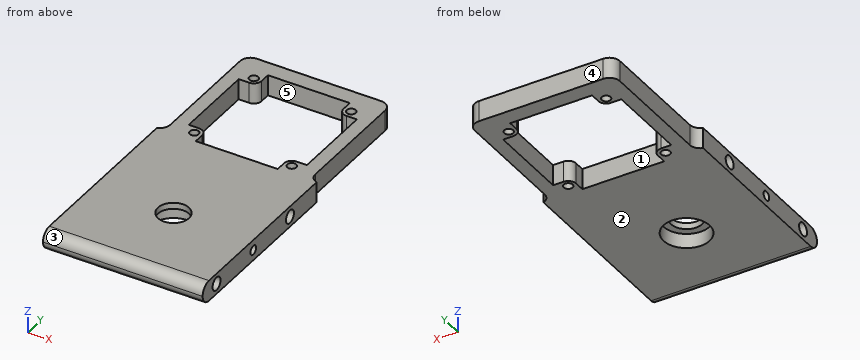
from build123d import *

# Parameters (mm, degrees)
AUFSATZ_LINEAR_AUSTRAGEN1_DEPTH  = 5
SKIZZE2_R                        = 3.15
SCHNITT_LINEAR_AUSTRAGEN1_DEPTH  = 139.488266651
SKIZZE3_R                        = 2.2
SCHNITT_LINEAR_AUSTRAGEN2_DEPTH  = 15
VERRUNDUNG2_R                    = 5
SCHNITT_LINEAR_AUSTRAGEN3_DEPTH  = 122.685044274
F_4_3_4_3_DURCHMESSER_BOHRUNG1_D = 4.3
VERRUNDUNG3_R                    = 5
VERRUNDUNG4_R                    = 5
SKIZZE8_R                        = 11.1
SCHNITT_LINEAR_AUSTRAGEN4_DEPTH  = 7
SKIZZE9_R                        = 7.5
SCHNITT_LINEAR_AUSTRAGEN5_DEPTH  = 10


# Some blends are built 0.0001 mm under size
with BuildPart() as part:
    # Skizze1 → Aufsatz-Linear austragen1 (new, symmetric)
    with BuildSketch(Plane.XY):
        Polygon((38.5, 50), (35, 50), (35, 115), (-35, 115), (-35, 50), (-38.5, 50), (-38.5, -40), (38.5, -40), align=None)
    extrude(amount=AUFSATZ_LINEAR_AUSTRAGEN1_DEPTH, both=True)

    # Skizze2 → Schnitt-Linear austragen1 (cut, through all)
    with BuildSketch(Plane.ZY.offset(38.5)):
        with Locations(Location((0, 29, 0), (0, 0, 270))):
            Circle(SKIZZE2_R)
        with Locations(Location((0, -29, 0), (0, 0, 90))):
            Circle(SKIZZE2_R)
    extrude(amount=-SCHNITT_LINEAR_AUSTRAGEN1_DEPTH, mode=Mode.SUBTRACT)

    # Skizze3 → Schnitt-Linear austragen2 (cut)
    with BuildSketch(Plane.ZY.offset(38.5)):
        with Locations(Location((0, 0, 0), (0, 0, 270))):
            Circle(SKIZZE3_R)
    schnitt_linear_austragen2 = extrude(amount=-SCHNITT_LINEAR_AUSTRAGEN2_DEPTH, mode=Mode.SUBTRACT)

    # Spiegeln1: Schnitt-Linear austragen2 across plane
    add(schnitt_linear_austragen2.mirror(Plane(origin=(0, 0, 0), x_dir=(0, 0, 1), z_dir=(1, 0, 0))), mode=Mode.SUBTRACT)

    # Verrundung2
    verrundung2_edges = [part.edges().sort_by_distance(p)[0] for p in [
        (0, -40, -5),
        (0, -40, 5),
    ]]
    fillet(verrundung2_edges, radius=VERRUNDUNG2_R - 0.0001)  # a hair under: the kernel refuses the full size

    # Skizze5 → Schnitt-Linear austragen3 (cut, through all)
    with BuildSketch(Plane.XY.offset(5)):
        with BuildLine():
            Line((19.75, 102), (19.75, 107))
            Line((19.75, 107), (-19.75, 107))
            Line((-19.75, 107), (-19.75, 102))
            ThreePointArc((-19.75, 102), (-20.848349571, 99.348349571), (-23.5, 98.25))
            Line((-23.5, 98.25), (-28.5, 98.25))
            Line((-28.5, 98.25), (-28.5, 58.75))
            Line((-28.5, 58.75), (-23.5, 58.75))
            ThreePointArc((-23.5, 58.75), (-20.848349571, 57.651650429), (-19.75, 55))
            Line((-19.75, 55), (-19.75, 50))
            Line((-19.75, 50), (19.75, 50))
            Line((19.75, 50), (19.75, 55))
            ThreePointArc((19.75, 55), (20.848349571, 57.651650429), (23.5, 58.75))
            Line((23.5, 58.75), (28.5, 58.75))
            Line((28.5, 58.75), (28.5, 98.25))
            Line((28.5, 98.25), (23.5, 98.25))
            ThreePointArc((23.5, 98.25), (20.848349571, 99.348349571), (19.75, 102))
        make_face()
    extrude(amount=-SCHNITT_LINEAR_AUSTRAGEN3_DEPTH, mode=Mode.SUBTRACT)

    # Ø4.3 (4.3) Durchmesser Bohrung1 (through all)
    with Locations(Plane.XY.offset(5)):
        with Locations((-23.5, 102), (-23.5, 55), (23.5, 55), (23.5, 102)):
            Hole(F_4_3_4_3_DURCHMESSER_BOHRUNG1_D / 2)

    # Verrundung3
    verrundung3_edges = [part.edges().sort_by_distance(p)[0] for p in [
        (-35, 115, 0),
        (35, 115, 0),
    ]]
    fillet(verrundung3_edges, radius=VERRUNDUNG3_R)

    # Verrundung4
    # the kernel refuses this fillet: 5 mm, written as the material it adds along each edge
    with BuildSketch(Plane(origin=(35, 50, -5), x_dir=(0, 1, 0), z_dir=(0, 0, 1))) as verrundung4_piece_1:
        with BuildLine():
            CenterArc((4.769696007, -5), VERRUNDUNG4_R, 90, 72.542396876)
            Line((0, -3.5), (-0.09539392, -3.47))
            ThreePointArc((-0.09539392, -3.47), (-0.1, -1.75), (-0.1, 0))
            Line((-0.1, 0), (0, 0.1))
            Line((0, 0.1), (4.769696007, 0.1))
            Line((4.769696007, 0.1), (4.769696007, 0))
        make_face()
    extrude(amount=10)
    with BuildSketch(Plane(origin=(-35, 50, -5), x_dir=(0, 1, 0), z_dir=(0, 0, 1))) as verrundung4_piece_2:
        with BuildLine():
            CenterArc((4.769696007, 5), VERRUNDUNG4_R, 197.457603124, 72.542396876)
            Line((0, 3.5), (-0.09539392, 3.47))
            ThreePointArc((-0.09539392, 3.47), (-0.1, 1.75), (-0.1, 0))
            Line((-0.1, 0), (0, -0.1))
            Line((0, -0.1), (4.769696007, -0.1))
            Line((4.769696007, -0.1), (4.769696007, 0))
        make_face()
    extrude(amount=10)

    # Skizze8 → Schnitt-Linear austragen4 (cut)
    with BuildSketch(Plane.XY.offset(-5)):
        Circle(SKIZZE8_R)
    extrude(amount=SCHNITT_LINEAR_AUSTRAGEN4_DEPTH, mode=Mode.SUBTRACT)

    # Skizze9 → Schnitt-Linear austragen5 (cut)
    with BuildSketch(Plane(origin=(0, 0, 2), x_dir=(-1, 0, 0), z_dir=(0, 0, -1))):
        Circle(SKIZZE9_R)
    extrude(amount=-SCHNITT_LINEAR_AUSTRAGEN5_DEPTH, mode=Mode.SUBTRACT)


solid = part.part
Input: part model. Units: mm. Frame: model coordinates. Face numbers are marked on the shaded views. A direction names the side the tool comes from. Give positions to 0.01 mm unless a question says otherwise; leave off trailing zeros. Write each loop counter-clockwise with the first axis right and the second up, starting at its lowest first coordinate (ties: lowest second). Pieces come first, ordered by that corner, then holes. Notation, with made-up numbers: M 75.25,4.25 L 112.25,4.25 A23 cw 112.25,39.25 Z; hole C 47.25,-1 d6. An arc over 180 degrees is marked long. Write item = value, one per line. Start each with the question number.
1) Material intervals for line 1 along Z through (x, y) = (-3, -29); line 2 along X through (y, z) = (60, -4); line 3 along Y through (x, z) = (20.5, -1.75), sorted ascending. Write a range as [from, to].
2) Cut plane D-D on y = -29. Return the cut outline in (x, z).
3) Cut plane A-A on x = 14.5. Count the separate pieces of the cut face and the enclosed holes in it, then the cut area to 3 significant figures.
4) Cut plane B-B on y = 0. Return the cut outline in (x, z).
5) Reachability of the marked faces 4 and 5 from +Z, -Z, +X, -X, +Y, -Y: full face, straight path, thin tool, end or side. Return the list, or none.
6) Draft query along Y for the marked faces 1, 2 and 3. Return one class per face: +Y half, -Y half, draft (parallel to the pull), parting line (faces both ways), or undercut.
7) First-contact query: pin 1 Ø1.5 at (y, z) = (104, -2.5) entering from +X; pin 2 Ø5.5 at (y, z) = (-29, 0) entering from +X; pin 3 Ø3.5 at (y, z) = (0, 0) entering from +X; pin 4 Ø2.5 at (y, z) = (52, 0) entering from +X. Flat tips, straight axial feed; report the tip coordinate or a pass-through.
Solved:
q1.line_1 = [-5, -3.15], [3.15, 5]
q1.line_2 = [-35, -28.5], [28.5, 35]
q1.line_3 = [-39.68, -31.62], [-26.38, 26.38], [31.62, 57.25], [99.75, 115]
q2.outline = M -38.5,-5 L 38.5,-5 L 38.5,-3.15 L -38.5,-3.15 Z; M -38.5,3.15 L 38.5,3.15 L 38.5,5 L -38.5,5 Z
q3.separate_pieces = 2
q3.enclosed_holes = 2
q3.area = 907 mm2
q4.outline = M -38.5,-5 L -11.1,-5 L -11.1,2 L -7.5,2 L -7.5,5 L -38.5,5 L -38.5,2.2 L -23.5,2.2 L -23.5,-2.2 L -38.5,-2.2 Z; M 7.5,2 L 11.1,2 L 11.1,-5 L 38.5,-5 L 38.5,-2.2 L 23.5,-2.2 L 23.5,2.2 L 38.5,2.2 L 38.5,5 L 7.5,5 Z
q5.face_4 = +Z, -Z, +X, -X, +Y
q5.face_5 = +Z, -Z
q6.face_1 = undercut
q6.face_2 = draft
q6.face_3 = -Y half
q7.pin_1 = 35
q7.pin_2 = through
q7.pin_3 = 23.5
q7.pin_4 = 37.03
